The listing builds one solid part. Answer for the finished solid, in the listing's coordinates (mm). A direction names the side the tool comes from. Coordinates: 2 decimals unless noted, no trailing zeros. Loops run counter-clockwise (first coordinate to the right, second up) from the corner with the lowest first, then second, coordinate; pieces in that order, holes last. Notation, with made-up numbers: M -24.75,27 L 28.25,27 A25 cw 28.25,56 Z; hole C 29,-27.75 d10. An arc over 180 degrees is marked long. Return JSON: item names as keys, results as strings. Group by question number.
1. Section C-C (x = 17) is taken. Write down the section's boundary in (y, z).
2. Given P1, Ø6, axis at x = 28.5, z = 12.5, coming from the -Y side; P2, Ø10, axis at x = 15, y = -6, coming from the +Z side; P3, Ø4, axis at x = 42.5, y = 14.5, coming from the -Z side, each flat-ended and moving along its own axis, determine where each tip first touches the part or whether it passes through.
3. Section A-A (z = 0) is taken. Write down the section's boundary in (x, y), then the cut area to 3 significant figures.
4. Which of the six approach directions +Z, -Z, +X, -X, +Y, -Y give full straight-line access (tool end or side, diameter ignored) to faces 1 (the face through (30.115, 18.548, -4.119)), 2 (the face through (3, -18.1, 1.4)), 3 (the face through (0, 18.2, 10.3))?
5. Straight lines are drawn through the part: L1, parallel to Y at x = 3.3, z = 0; L2, parallel to Z at x = 45, y = 13; L3, parallel to Y at x = 36, z = 10. For each, find the intervals that lie inside material, in ascending order. Write a range as from..to.
```python
from build123d import *

# Parameters (mm, degrees)
SKETCH_2_R          = 20.5
CUT_EXTRUDE_1_DEPTH = 3
SKETCH_3_R          = 18
CUT_EXTRUDE_2_DEPTH = 0.5
CHAMFER_1_SIZE      = 0.5


with BuildPart() as part:
    # 스케치1 → 회전1 (revolve)
    with BuildSketch(Plane.XY, mode=Mode.PRIVATE) as revolve_1_sk:
        Polygon((0, 17.5), (0, 27.5), (4, 27.5), (7.093746991, 19), (53, 19), (53, 17.5), align=None)
    revolve(revolve_1_sk.sketch.rotate(Axis((0, 0, 0), (1, 0, 0)), 90), axis=Axis((0, 0, 0), (1, 0, 0)))

    # 스케치2 → 컷-돌출1 (cut)
    with BuildSketch(Plane.ZY):
        Circle(SKETCH_2_R)
    extrude(amount=-CUT_EXTRUDE_1_DEPTH, mode=Mode.SUBTRACT)

    # 스케치3 → 컷-돌출2 (cut)
    with BuildSketch(Plane.ZY.offset(-3)):
        Circle(SKETCH_3_R)
    extrude(amount=-CUT_EXTRUDE_2_DEPTH, mode=Mode.SUBTRACT)

    # 모따기1
    chamfer_1_edges = [part.edges().sort_by_distance(p)[0] for p in [
        (53, 0, -19),
    ]]
    chamfer(chamfer_1_edges, length=CHAMFER_1_SIZE)


solid = part.part
```
Worked out:
{
 "1": {"outline": "C 0,0 d38; hole C 0,0 d35"},
 "2": {"P1": "y = -16.45", "P2": "z = 18.97", "P3": "z = -14.31"},
 "3": {"outline": "M 0,-27.5 L 4,-27.5 L 7.09,-19 L 52.5,-19 L 53,-18.5 L 53,-17.5 L 3.5,-17.5 L 3.5,-18 L 3,-18 L 3,-20.5 L 0,-20.5 Z; M 0,20.5 L 3,20.5 L 3,18 L 3.5,18 L 3.5,17.5 L 53,17.5 L 53,18.5 L 52.5,19 L 7.09,19 L 4,27.5 L 0,27.5 Z", "area": "235 mm^2"},
 "4": {"face 1": "+X", "face 2": "-X", "face 3": "+Z, -Z, -X, +Y, -Y"},
 "5": {"L1": "-27.5..-18, 18..27.5", "L2": "-13.86..-11.72, 11.72..13.86", "L3": "-16.16..-14.36, 14.36..16.16"}
}
